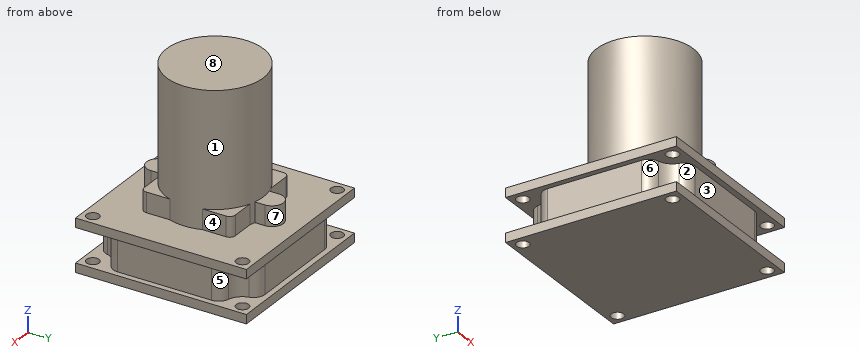
Autodesk Inventor part; units mm, degrees
ref_plane "作業平面1" through (0, 0, 27.5) normal (0, 0, 1) x (1, 0, 0)
ref_plane "YZ Plane" through (0, 0, 0) normal (1, 0, 0) x (0, 1, 0)
ref_plane "XZ Plane" through (0, 0, 0) normal (0, 1, 0) x (-1, 0, 0)
sketch "スケッチ1" plane through (0, 0, 0) normal (0, 0, 1) x (1, 0, 0)
  line L0 (-15, -15) -> (15, -15)
  line L1 (15, -15) -> (15, 15)
  line L2 (15, 15) -> (-15, 15)
  line L3 (-15, 15) -> (-15, -15)
  line L4 (-15, -15) -> (15, 15) construction
  line L5 (15, -15) -> (-15, 15) construction
  line L6 (-15, 0) -> (15, 0) construction
  line L7 (0, 15) -> (0, -15) construction
  line L8 (-13.14, 13.14) -> (13.14, 13.14) construction
  line L9 (13.14, 13.14) -> (13.14, -13.14) construction
  line L10 (13.14, -13.14) -> (-13.14, -13.14) construction
  line L11 (-13.14, -13.14) -> (-13.14, 13.14) construction
  line L12 (-13.14, 13.14) -> (13.14, -13.14) construction
  line L13 (13.14, 13.14) -> (-13.14, -13.14) construction
  circle A0 centre (0, 0) radius 8.5
  line L14 (-7, 8) -> (7, 8)
  line L15 (8, 7) -> (8, -7)
  line L16 (7, -8) -> (-7, -8)
  line L17 (-8, -7) -> (-8, 7)
  line L18 (-8, 8) -> (8, -8) construction
  line L19 (8, 8) -> (-8, -8) construction
  arc A1 (-8, -7) -> (-7, -8) centre (-7, -7) ccw
  arc A2 (7, -8) -> (8, -7) centre (7, -7) ccw
  arc A3 (8, 7) -> (7, 8) centre (7, 7) ccw
  arc A4 (-7, 8) -> (-8, 7) centre (-7, 7) ccw
  arc A5 (-2, -10) -> (2, -10) centre (0, -10) ccw
  line L20 (-2, -10) -> (-2, -8)
  line L21 (2, -10) -> (2, -8)
  arc A6 (2, 10) -> (-2, 10) centre (0, 10) ccw
  line L22 (-2, 10) -> (-2, 8)
  line L23 (2, 10) -> (2, 8)
  circle A7 centre (-13.14, -13.14) radius 1.1
  circle A8 centre (13.14, -13.14) radius 1.1
  circle A9 centre (-13.14, 13.14) radius 1.1
  circle A10 centre (13.14, 13.14) radius 1.1
  circle A11 centre (-13.14, -13.14) radius 2 construction
  circle A12 centre (13.14, -13.14) radius 2 construction
  circle A13 centre (-13.14, 13.14) radius 2 construction
  circle A14 centre (13.14, 13.14) radius 2 construction
  arc A15 (-10.219, -12.456) -> (-12.456, -10.219) centre (-13.14, -13.14) ccw
  line L24 (-14, -8.2717) -> (-14, 8.2717)
  line L25 (-8.2717, -14) -> (8.2717, -14)
  arc A16 (-14, -8.2717) -> (-12.456, -10.219) centre (-12, -8.2717) ccw
  arc A17 (-10.219, -12.456) -> (-8.2717, -14) centre (-8.2717, -12) ccw
  arc A18 (-12.456, 10.219) -> (-10.219, 12.456) centre (-13.14, 13.14) ccw
  line L26 (-8.2717, 14) -> (8.2717, 14)
  arc A19 (-12.456, 10.219) -> (-14, 8.2717) centre (-12, 8.2717) ccw
  arc A20 (-8.2717, 14) -> (-10.219, 12.456) centre (-8.2717, 12) ccw
  arc A21 (12.456, -10.219) -> (10.219, -12.456) centre (13.14, -13.14) ccw
  line L27 (14, -8.2717) -> (14, 8.2717)
  arc A22 (12.456, -10.219) -> (14, -8.2717) centre (12, -8.2717) ccw
  arc A23 (8.2717, -14) -> (10.219, -12.456) centre (8.2717, -12) ccw
  arc A24 (14, 8.2717) -> (12.456, 10.219) centre (12, 8.2717) ccw
  arc A25 (10.219, 12.456) -> (12.456, 10.219) centre (13.14, 13.14) ccw
  arc A26 (10.219, 12.456) -> (8.2717, 14) centre (8.2717, 12) ccw
  point P0 (-10.2659, -14)
  point P1 (-14, -10.2659)
  point P2 (-8, -2.8723)
  point P3 (-8, 2.8723)
  point P4 (-2.8723, 8)
  point P5 (-2, 8.2614)
  point P6 (2, 8.2614)
  point P7 (2.8723, 8)
  point P8 (8, 2.8723)
  point P9 (8, -2.8723)
  point P10 (2.8723, -8)
  point P11 (2, -8.2614)
  point P12 (-2, -8.2614)
  point P13 (-2.8723, -8)
  dimension "d0" = 30
  dimension "d1" = 30
  dimension "d2" = 26.28
  dimension "d3" = 26.28
  dimension "d4" = 17
  dimension "d5" = 16
  dimension "d6" = 16
  dimension "d7" = 1
  dimension "d8" = 20
  dimension "d9" = 2
  dimension "d10" = 2.2
  dimension "d11" = 4
  dimension "d12" = 2
  dimension "d13" = 3
  dimension "d14" = 1
  dimension "d15" = 1
extrude "押し出し1" add sketch "スケッチ1" along normal blind 9.2 contours L3 L2 L1 L0 | A15 A16 L24 A19 A18 A20 L26 A26 A25 A24 L27 A22 A21 A23 L25 A17
extrude "押し出し2" cut sketch "スケッチ1" along normal blind 7.6 contours L3 L2 L1 L0
extrude "押し出し3" add sketch "スケッチ1" along normal blind 1.6 contours L3 L2 L1 L0
extrude "押し出し4" add sketch "スケッチ1" along normal blind 12.7 contours A0 L14 A3 L15 | L15 A2 L16 A0 | A0 L22 A6 L23 | L21 A5 L20 A0 | A0 L17 A4 L14 | L16 A1 L17 A0
extrude "押し出し5" add sketch "スケッチ1" along normal blind 32.8 contours A0 L15 | L15 A0 L16 L17 L14 | L14 L23 A0 | A0 L21 L16 | L23 L14 L22 A0 | A0 L20 L16 L21 | L22 L14 A0 | A0 L16 L20 | L17 A0
ref_plane "作業平面1" through (0, 0, 27.5) normal (0, 0, 1) x (1, 0, 0)
sketch "focus of the lens" plane through (0, 0, 27.5) normal (0, 0, 1) x (1, 0, 0)
  point P0 (0, 0)
  point P1 (0, 0)
equation "\"d1\" = d0"
equation "\"d3\" = d2"
equation "\"d6\" = d5"
equation "\"d15\" = d14"
properties part number "e-CAM50_CUNX"
Geometry: final body of the model. Coordinates: model frame, mm. Face numbers are marked on the shaded views. A direction names the side the tool comes from. Round coordinates to 2 decimals unless told otherwise and drop trailing zeros. Loops run counter-clockwise (first coordinate to the right, second up) from the corner with the lowest first, then second, coordinate; pieces in that order, holes last. Notation, with made-up numbers: (39.25, 52) -> (83.25, 52) arc R12 cw to (83.25, 64) -> close; hole circle Ø4 at (59, 68.25). An arc over 180 degrees is marked (long way). One line per question, with ' | ' between items. Start each with the question number.
1. Mould query, pull axis Z, two halves, no side actions, for the marked faces 6, 7 and 8. Classes: pulls with the +Z half, pulls with the -Z half, needs draft (parallel to the pull), parting line crosses it, or undercut.
2. Section B-B on y = -13.14. Output: boundary loops of the cut face in (x, z).
3. Line query: line 1 along Y through (x, z) = (13.14, 8.05); line 2 along Z through (x, y) = (11, -13); line 3 along Z through (x, y) = (-9.5, 11.5). Output: solid intervals per line, ascending. Write a range as [from, to].
4. Section D-D on z = 4.5. Output: boundary loops of the cut face in (x, y).
5. Section C-C on x = -5.75. Output: boundary loops of the cut face in (y, z).
6. Set-up query: the marked faces 1, 2, 3, 4 and 5. Return all of +Z, -Z, +X, -X, +Y, -Y with unobstructed straight access to the full face (end or side cutting, diameter ignored); none if empty.
7. Section A-A on z = 8.5. Output: boundary loops of the cut face in (x, y), and give its area (3 significant figures).
8. Contact query for flat-ended pins moving along their axis: pin 1 (3.5 mm diameter, centred on x = -13.14, y = 13.14, fed in from +Z); pin 2 (5 mm diameter, centred on y = 7.5, z = 20, fed in from +X); pin 3 (4 mm diameter, centred on y = 8, z = 23, fed in from +X); pin 4 (1.3 mm diameter, centred on x = 13.14, y = 13.14, fed in from +Z). Output: stop coordinate, or through.
Returned:
1) face 6: undercut | face 7: needs draft | face 8: pulls with the +Z half
2) outline: (-15, 0) -> (-14.24, 0) -> (-14.24, 1.6) -> (-15, 1.6) -> close; (-15, 7.6) -> (-14.24, 7.6) -> (-14.24, 9.2) -> (-15, 9.2) -> close; (-12.04, 0) -> (12.04, 0) -> (12.04, 1.6) -> (9.91, 1.6) -> (9.91, 7.6) -> (12.04, 7.6) -> (12.04, 9.2) -> (-12.04, 9.2) -> (-12.04, 7.6) -> (-9.91, 7.6) -> (-9.91, 1.6) -> (-12.04, 1.6) -> close; (14.24, 0) -> (15, 0) -> (15, 1.6) -> (14.24, 1.6) -> close; (14.24, 7.6) -> (15, 7.6) -> (15, 9.2) -> (14.24, 9.2) -> close
3) line 1: y = [-15, -14.24], [-12.04, 12.04], [14.24, 15] | line 2: z = [0, 1.6], [7.6, 9.2] | line 3: z = [0, 9.2]
4) outline: (-14, -8.27) arc R2 ccw to (-12.46, -10.22) arc R3 cw to (-10.22, -12.46) arc R2 ccw to (-8.27, -14) -> (8.27, -14) arc R2 ccw to (10.22, -12.46) arc R3 cw to (12.46, -10.22) arc R2 ccw to (14, -8.27) -> (14, 8.27) arc R2 ccw to (12.46, 10.22) arc R3 cw to (10.22, 12.46) arc R2 ccw to (8.27, 14) -> (-8.27, 14) arc R2 ccw to (-10.22, 12.46) arc R3 cw to (-12.46, 10.22) arc R2 ccw to (-14, 8.27) -> close
5) outline: (-15, 0) -> (15, 0) -> (15, 1.6) -> (14, 1.6) -> (14, 7.6) -> (15, 7.6) -> (15, 9.2) -> (8, 9.2) -> (8, 12.7) -> (6.26, 12.7) -> (6.26, 32.8) -> (-6.26, 32.8) -> (-6.26, 12.7) -> (-8, 12.7) -> (-8, 9.2) -> (-15, 9.2) -> (-15, 7.6) -> (-14, 7.6) -> (-14, 1.6) -> (-15, 1.6) -> close
6) face 1: +Z | face 2: -X, -Y | face 3: +X, -X, -Y | face 4: +Z, +X, +Y | face 5: +X, +Y
7) outline: (-15, -15) -> (15, -15) -> (15, 15) -> (-15, 15) -> close; hole circle Ø2.2 at (-13.14, -13.14); hole circle Ø2.2 at (-13.14, 13.14); hole circle Ø2.2 at (13.14, -13.14); hole circle Ø2.2 at (13.14, 13.14) | area: 885 mm2
8) pin 1: stops at z = 9.2 | pin 2: stops at x = 6.87 | pin 3: stops at x = 6.02 | pin 4: passes through
